Geometry check sheet. Reference: the model listing, model coordinates, mm. Face numbers are marked on the shaded views. A direction names the side the tool comes from. Round coordinates to 2 decimals unless told otherwise and drop trailing zeros. Loops run counter-clockwise (first coordinate to the right, second up) from the corner with the lowest first, then second, coordinate; pieces in that order, holes last. Notation, with made-up numbers: (21.5, 63) -> (62.5, 63) arc R7 ccw to (62.5, 73) -> close; hole circle Ø4 at (-14, -25). An arc over 180 degrees is marked (long way). Use a Markdown table: item, result. Add a question column.
Q1. Sectioned sample at B-B, the plane x = 7.5. Enter the section's corners in (y, z), then the cut area to 3 significant figures.
Q2. Sectioned sample at A-A, the plane y = -590. Enter the section's corners in (x, z).
Q3. Gauge pin test, flat ends, axial feed: P1, Ø1, axis at y = -632.5, z = 25.5, coming from the +X side; P2, Ø1, axis at x = 24, y = -1545.5, coming from the +Z side. Record the tip position at first contact, or that the pin passes through.
Q4. Set-up check for the marked faces 1 and 2: record each of +Z, -Z, +X, -X, +Y, -Y from which the full face is reachable in a straight line by a thin tool's end or side.
Q5. Material ranges on L1, parallel to Z at x = 32, y = -2020; L2, parallel to Z at x = -33, y = -701.5; L3, parallel to X at y = -797, z = -29.5, recorded low to high.
Q6. Sectioned sample at C-C, the plane z = -2.5. Enter the section's corners in (x, y), then the cut area to 3 significant figures.
```python
from build123d import *

# Parameters (mm, degrees)
F1_DEPTH = 2133.6


with BuildPart() as f1:
    # F0 (on Front) → F1 (new body)
    with BuildSketch(Plane.XZ):
        with BuildLine():
            Line((-44.45, -38.1), (-44.45, 0))
            Line((-44.45, 0), (-63.5, 0))
            Line((-63.5, 0), (-63.5, -44.45))
            Line((-63.5, -44.45), (-63.5, -69.85))
            Line((-63.5, -69.85), (-44.45, -69.85))
            Line((-44.45, -69.85), (63.5, -69.85))
            Line((63.5, -69.85), (63.5, -57.15))
            ThreePointArc((63.5, -57.15), (61.640128, -52.659872), (57.15, -50.8))
            Line((57.15, -50.8), (-31.75, -50.8))
            ThreePointArc((-31.75, -50.8), (-40.730256, -47.080256), (-44.45, -38.1))
        make_face()
        with BuildLine():
            Line((-63.5, 0), (-44.45, 0))
            Line((-44.45, 0), (-44.45, 57.15))
            ThreePointArc((-44.45, 57.15), (-46.309872, 61.640128), (-50.8, 63.5))
            Line((-50.8, 63.5), (-63.5, 63.5))
            Line((-63.5, 63.5), (-63.5, 0))
        make_face()
    extrude(amount=F1_DEPTH)


solid = f1.part
```
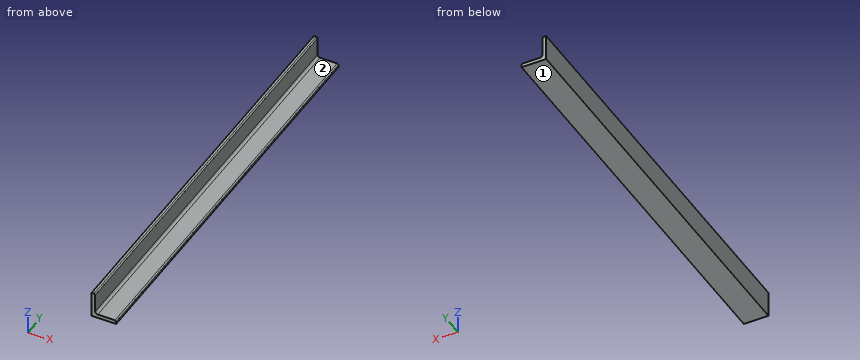
Values:
| question | item | result |
|---|---|---|
| 1 | outline | (-2133.6, -69.85) -> (0, -69.85) -> (0, -50.8) -> (-2133.6, -50.8) -> close |
| 1 | area | 40,600 mm^2 |
| 2 | outline | (-63.5, -69.85) -> (63.5, -69.85) -> (63.5, -57.15) arc R6.35 ccw to (57.15, -50.8) -> (-31.75, -50.8) arc R12.7 cw to (-44.45, -38.1) -> (-44.45, 57.15) arc R6.35 ccw to (-50.8, 63.5) -> (-63.5, 63.5) -> close |
| 3 | P1 | x = -44.45 |
| 3 | P2 | z = -50.8 |
| 4 | face 1 | -Z, +X, -X, +Y, -Y |
| 4 | face 2 | +Z, +X, +Y, -Y |
| 5 | L1 | -69.85 to -50.8 |
| 5 | L2 | -69.85 to -50.74 |
| 5 | L3 | -63.5 to -44.45 |
| 6 | outline | (-63.5, -2133.6) -> (-44.45, -2133.6) -> (-44.45, 0) -> (-63.5, 0) -> close |
| 6 | area | 40,600 mm^2 |
